Model file for the job. Use its own axes, mm. Give positions to 0.01 mm unless a question says otherwise; leave off trailing zeros. Loops run counter-clockwise (first coordinate to the right, second up) from the corner with the lowest first, then second, coordinate; pieces in that order, holes last. Notation, with made-up numbers: M -38,52 L -9,52 A19 ccw -9,68 Z; hole C -1,-13.5 d2. An arc over 180 degrees is marked long. Answer in a Markdown table with one row per item.
```python
from build123d import *

# Parameters (mm, degrees)
SKETCH1_R           = 47.5
BOSS_EXTRUDE1_DEPTH = 62
SKETCH2_W           = 10
SKETCH2_H           = 5
CUT_EXTRUDE1_DEPTH  = 20
SKETCH3_R           = 5
CUT_EXTRUDE2_DEPTH  = 63


with BuildPart() as part:
    # Sketch1 → Boss-Extrude1 (new body)
    with BuildSketch(Plane.XY):
        Circle(SKETCH1_R)
    extrude(amount=BOSS_EXTRUDE1_DEPTH)

    # Sketch2 → Cut-Extrude1 (cut)
    with BuildSketch(Plane.XY.offset(62)):
        with Locations((10, 0)):
            Rectangle(SKETCH2_W, SKETCH2_H)
    extrude(amount=-CUT_EXTRUDE1_DEPTH, mode=Mode.SUBTRACT)

    # Sketch3 → Cut-Extrude2 (cut, through all)
    with BuildSketch(Plane.XY.offset(62)):
        with Locations((0, 32.5)):
            Circle(SKETCH3_R)
        with Locations((28.145825623, -16.25)):
            Circle(SKETCH3_R)
        with Locations((-28.145825623, -16.25)):
            Circle(SKETCH3_R)
    extrude(amount=-CUT_EXTRUDE2_DEPTH, mode=Mode.SUBTRACT)


solid = part.part
```
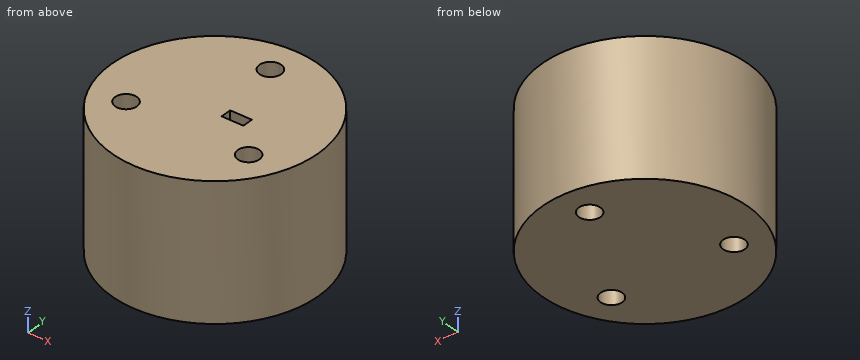
Q1. Saw through at C-C (y = -16.25). Give the cut face in (x, z).
Reported:
| item | result |
|---|---|
| outline | M -44.63,0 L -33.15,0 L -33.15,62 L -44.63,62 Z; M -23.15,0 L 23.15,0 L 23.15,62 L -23.15,62 Z; M 33.15,0 L 44.63,0 L 44.63,62 L 33.15,62 Z |
Q2. Saw through at D-D (z = 17.5). Give the cut face in (x, y), and give its area (3 significant figures).
Reported:
| item | result |
|---|---|
| outline | C 0,0 d95; hole C -28.15,-16.25 d10; hole C 0,32.5 d10; hole C 28.15,-16.25 d10 |
| area | 6,850 mm² |
Q3. Drop flat-ended pins along their axis: pin 1 (8 mm diameter, centred on x = -32.5, z = 23.5, fed in from +Y); pin 2 (8 mm diameter, centred on x = 10.5, z = 48, fed in from -Y); pin 3 (6 mm diameter, centred on x = 28.15, y = -16.25, fed in from +Z); pin 4 (12 mm diameter, centred on x = 2.5, z = 52.5, fed in from +Y). Give the stop position or say it passes through.
Reported:
| item | result |
|---|---|
| pin 1 | y = 38 |
| pin 2 | y = -47.05 |
| pin 3 | through |
| pin 4 | y = 47.5 |
Q4. Saw through at A-A (x = 0). Give the cut face in (y, z), and give its area (3 significant figures).
Reported:
| item | result |
|---|---|
| outline | M -47.5,0 L 27.5,0 L 27.5,62 L -47.5,62 Z; M 37.5,0 L 47.5,0 L 47.5,62 L 37.5,62 Z |
| area | 5,270 mm² |
Q5. Saw through at B-B (y = 32.5). Give the cut face in (x, z).
Reported:
| item | result |
|---|---|
| outline | M -34.64,0 L -5,0 L -5,62 L -34.64,62 Z; M 5,0 L 34.64,0 L 34.64,62 L 5,62 Z |
Q6. Probe probe 1 along Y at (x, z) = (0, 53); probe 2 along X at (y, z) = (32, 23); probe 3 along Y at (x, z) = (-30.5, 55). List the from-to ranges inside material, lowest first.
Reported:
| item | result |
|---|---|
| probe 1 | -47.5 to 27.5, 37.5 to 47.5 |
| probe 2 | -35.1 to -4.97, 4.97 to 35.1 |
| probe 3 | -36.41 to -20.66, -11.84 to 36.41 |
